Could you check a few things on this model? Use its own coordinates, in mm. Face numbers are marked on the shaded views. A direction names the side the tool comes from. Give positions to 0.01 mm unless a question says otherwise; leave off trailing zeros. Write each loop counter-clockwise with the first axis right and the second up, starting at its lowest first coordinate (ties: lowest second). Pieces come first, ordered by that corner, then holes. Notation, with made-up numbers: (-10.5, -14) - (0.5, -14) arc R31 ccw to (0.5, 21) - close; hole circle Ø1 at (-19, 7). An arc over 180 degrees is marked (long way). Answer as CSV lines item,"result". Start each with the question number.
Q1. On a 3-axis mill with a long thin cutter (end or side, diameter ignored), from which of +Z, -Z, +X, -X, +Y, -Y can I reach the whole of each face in a straight line? I mean the marked faces 1, 2 and 3. Say none if no direction works.
Q2. If I drill on line 1 along Y through (x, z) = (-13.75, 67.1); line 2 along X through (y, z) = (7, 43); line 3 along Z through (x, y) = (-3, -14.5), over which ranges is the centre line in solid material (lowest first)?
Q3. Imagine slicing it at C-C on y = -30.16. List the corners of the cut face in (x, z) for me, and give its area (3 significant figures).
Q4. Imagine slicing it at B-B on z = 67.1. List the corners of the cut face in (x, y) for me.
Q5. Will these pins go through, and if not, where does the flat tip stop? pin 1 Ø0.7 at (y, z) = (-14.5, 21) entering from +X; pin 2 Ø0.5 at (x, z) = (5, 0) entering from -Y; pin 3 Ø8 at (x, y) = (-2, -7.5) entering from +Z; pin 4 Ø2.5 at (y, z) = (2.34, 49.9) entering from -X.
Q6. Imagine slicing it at D-D on z = 30.5. List the corners of the cut face in (x, y) for me, and give its area (3 significant figures).
Q7. Imagine slicing it at A-A on y = 2.34. List the corners of the cut face in (x, z) for me.
```python
from build123d import *

# Parameters (mm, degrees)
SKETCH1_W                    = 28.1256
SKETCH1_H                    = 30
BASE_FLANGE2_DEPTH           = 0.8128
EDGE_FLANGE3_STRIP_W         = 4.7244
EDGE_FLANGE3_STRIP_H         = 0.8128
EDGE_FLANGE3_STRIP_CUT_DEPTH = 30
EDGE_FLANGE3_DEPTH           = 30
EDGE_FLANGE3_FLAT_DEPTH      = 0.8128
EDGE_FLANGE4_START           = 0.7366
EDGE_FLANGE4_DEPTH           = 56.7698
EDGE_FLANGE4_START_2         = 57.1
EDGE_FLANGE4_2_DEPTH         = 0.4064
EDGE_FLANGE4_3_DEPTH         = 56.3634
CUT_EXTRUDE1_REACH           = 93.299
SKETCH22_R                   = 2
CUT_EXTRUDE2_REACH           = 89.146


# Read off the part's stored shape, not the designer's step: Edge-Flange4
# Sheet-metal steps are written as plain solids
with BuildPart() as part:
    # Sketch1 → Base-Flange2 (new body)
    with BuildSketch(Plane.XY):
        Rectangle(SKETCH1_W, SKETCH1_H)
    extrude(amount=-BASE_FLANGE2_DEPTH)

    # Edge-Flange3 strip (across the edge) → Edge-Flange3 strip cut (cut)
    with BuildSketch(Plane(origin=(-14.0628, 15, 0), x_dir=(1, 0, 0), z_dir=(0, -1, 0))):
        with Locations((-0.8128, -0.4064)):
            Rectangle(EDGE_FLANGE3_STRIP_W, EDGE_FLANGE3_STRIP_H)
    extrude(amount=EDGE_FLANGE3_STRIP_CUT_DEPTH, mode=Mode.SUBTRACT)

    # Edge-Flange3 bend section (across the edge) → Edge-Flange3 (add)
    with BuildSketch(Plane(origin=(-14.0628, 15, 0), x_dir=(1, 0, 0), z_dir=(0, -1, 0))):
        with BuildLine():
            Line((0, 0.7366), (0.8128, 0.7366))
            ThreePointArc((0.8128, 0.7366), (1.028545145, 0.215745145), (1.5494, 0))
            Line((1.5494, 0), (1.5494, -0.8128))
            ThreePointArc((1.5494, -0.8128), (0.453808753, -0.358991247), (0, 0.7366))
        make_face()
    extrude(amount=EDGE_FLANGE3_DEPTH)

    # Edge-Flange3 profile (on flange) → Edge-Flange3 flat (add)
    with BuildSketch(Plane(origin=(-14.0628, 0, 0), x_dir=(0, -1, 0), z_dir=(-1, 0, 0))):
        Polygon((-15, 0.7366), (15, 0.7366), (15, 57.1), (40, 57.1), (40, 77.1), (-15, 77.1), align=None)
    extrude(amount=-EDGE_FLANGE3_FLAT_DEPTH)

    # Edge-Flange4 outline → Edge-Flange4 (cut)
    with BuildSketch(Plane.XY.offset(EDGE_FLANGE4_START)):
        with BuildLine():
            ThreePointArc((-13.25, -13.4506), (-13.468624211, -14.244121367), (-14.0628, -14.813707039))
            Line((-14.0628, -14.813707039), (-14.0628, -15))
            Line((-14.0628, -15), (-13.25, -15))
            Line((-13.25, -15), (-13.25, -13.4506))
        make_face()
    extrude(amount=EDGE_FLANGE4_DEPTH, mode=Mode.SUBTRACT)

    # Edge-Flange4 2 outline → Edge-Flange4 2 (cut)
    with BuildSketch(Plane.XY.offset(EDGE_FLANGE4_START_2)):
        with BuildLine():
            Line((-14.0628, -13.0442), (-14.0628, -14.813707039))
            ThreePointArc((-14.0628, -14.813707039), (-13.468624211, -14.244121367), (-13.25, -13.4506))
            Line((-13.25, -13.4506), (-13.25, -13.0442))
            Line((-13.25, -13.0442), (-14.0628, -13.0442))
        make_face()
    extrude(amount=EDGE_FLANGE4_2_DEPTH, mode=Mode.SUBTRACT)

    # Edge-Flange4 3 outline → Edge-Flange4 3 (add)
    with BuildSketch(Plane.XY.offset(EDGE_FLANGE4_START)):
        with BuildLine():
            Line((-28.25, -15), (-14.7994, -15))
            ThreePointArc((-14.7994, -15), (-14.419503755, -14.952704924), (-14.0628, -14.813707039))
            Line((-14.0628, -14.813707039), (-14.0628, -13.4506))
            ThreePointArc((-14.0628, -13.4506), (-14.278545145, -13.971454855), (-14.7994, -14.1872))
            Line((-14.7994, -14.1872), (-28.25, -14.1872))
            Line((-28.25, -14.1872), (-28.25, -15))
        make_face()
    extrude(amount=EDGE_FLANGE4_3_DEPTH)

    # Sketch22 → Cut-Extrude1 (cut, up to next)
    with BuildSketch(Plane.ZY.offset(14.0628), mode=Mode.PRIVATE) as cut_extrude1_sk1:
        with Locations((67.1, -30.16)):
            Circle(SKETCH22_R)
    cut_extrude1_tool1 = extrude(cut_extrude1_sk1.sketch, amount=-CUT_EXTRUDE1_REACH, mode=Mode.PRIVATE) & part.part
    # Sketch22 → Cut-Extrude1 (cut, up to next)
    with BuildSketch(Plane.ZY.offset(14.0628), mode=Mode.PRIVATE) as cut_extrude1_sk2:
        with Locations((67.1, -7.66)):
            Circle(SKETCH22_R)
    cut_extrude1_tool2 = extrude(cut_extrude1_sk2.sketch, amount=-CUT_EXTRUDE1_REACH, mode=Mode.PRIVATE) & part.part
    # Sketch22 → Cut-Extrude1 (cut, up to next)
    with BuildSketch(Plane.ZY.offset(14.0628), mode=Mode.PRIVATE) as cut_extrude1_sk3:
        with Locations((49.895058849, 2.34)):
            Circle(SKETCH22_R)
    cut_extrude1_tool3 = extrude(cut_extrude1_sk3.sketch, amount=-CUT_EXTRUDE1_REACH, mode=Mode.PRIVATE) & part.part
    # Sketch22 → Cut-Extrude1 (cut, up to next)
    with BuildSketch(Plane.ZY.offset(14.0628), mode=Mode.PRIVATE) as cut_extrude1_sk4:
        with Locations((29.995058849, 2.34)):
            Circle(SKETCH22_R)
    cut_extrude1_tool4 = extrude(cut_extrude1_sk4.sketch, amount=-CUT_EXTRUDE1_REACH, mode=Mode.PRIVATE) & part.part
    # Sketch22 → Cut-Extrude1 (cut, up to next)
    with BuildSketch(Plane.ZY.offset(14.0628), mode=Mode.PRIVATE) as cut_extrude1_sk5:
        with Locations((10.095058849, 2.34)):
            Circle(SKETCH22_R)
    cut_extrude1_tool5 = extrude(cut_extrude1_sk5.sketch, amount=-CUT_EXTRUDE1_REACH, mode=Mode.PRIVATE) & part.part
    add(cut_extrude1_tool1.solids().sort_by_distance((-14.0628, -30.16, 67.1))[0], mode=Mode.SUBTRACT)
    add(cut_extrude1_tool2.solids().sort_by_distance((-14.0628, -7.66, 67.1))[0], mode=Mode.SUBTRACT)
    add(cut_extrude1_tool3.solids().sort_by_distance((-14.0628, 2.34, 49.895059))[0], mode=Mode.SUBTRACT)
    add(cut_extrude1_tool4.solids().sort_by_distance((-14.0628, 2.34, 29.995059))[0], mode=Mode.SUBTRACT)
    add(cut_extrude1_tool5.solids().sort_by_distance((-14.0628, 2.34, 10.095059))[0], mode=Mode.SUBTRACT)

    # Sketch23 → Cut-Extrude2 (cut, up to next)
    with BuildSketch(Plane(origin=(0, -14.1872, 0), x_dir=(1, 0, 0), z_dir=(0, 1, 0)), mode=Mode.PRIVATE) as cut_extrude2_sk1:
        with BuildLine():
            Line((-26.8128, -26.4866), (-26.8128, -18.4866))
            ThreePointArc((-26.8128, -18.4866), (-24.0628, -15.7366), (-21.3128, -18.4866))
            Line((-21.3128, -18.4866), (-21.3128, -26.4866))
            ThreePointArc((-21.3128, -26.4866), (-24.0628, -29.2366), (-26.8128, -26.4866))
        make_face()
    cut_extrude2_tool1 = extrude(cut_extrude2_sk1.sketch, amount=-CUT_EXTRUDE2_REACH, mode=Mode.PRIVATE) & part.part
    # Sketch23 → Cut-Extrude2 (cut, up to next)
    with BuildSketch(Plane(origin=(0, -14.1872, 0), x_dir=(1, 0, 0), z_dir=(0, 1, 0)), mode=Mode.PRIVATE) as cut_extrude2_sk2:
        with BuildLine():
            Line((-26.8128, -41.9866), (-26.8128, -49.9866))
            ThreePointArc((-26.8128, -49.9866), (-24.0628, -52.7366), (-21.3128, -49.9866))
            Line((-21.3128, -49.9866), (-21.3128, -41.9866))
            ThreePointArc((-21.3128, -41.9866), (-24.0628, -39.2366), (-26.8128, -41.9866))
        make_face()
    cut_extrude2_tool2 = extrude(cut_extrude2_sk2.sketch, amount=-CUT_EXTRUDE2_REACH, mode=Mode.PRIVATE) & part.part
    add(cut_extrude2_tool1.solids().sort_by_distance((-24.0628, -14.1872, 22.4866))[0], mode=Mode.SUBTRACT)
    add(cut_extrude2_tool2.solids().sort_by_distance((-24.0628, -14.1872, 45.9866))[0], mode=Mode.SUBTRACT)


solid = part.part
```
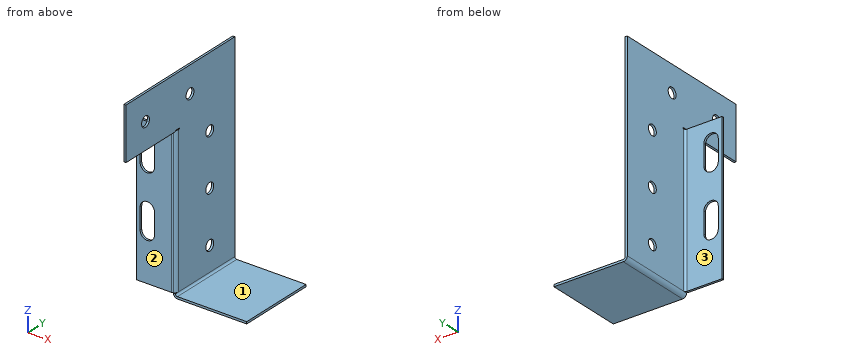
Conclusion:
1,face 1,"+Z, +X, +Y, -Y"
1,face 2,"+Z, -Z, +X, -X, -Y"
1,face 3,"+Z, -Z, -X, +Y"
2,line 1,"-40 to -32.16, -28.16 to -9.66, -5.66 to 15"
2,line 2,"-14.06 to -13.25"
2,line 3,"-0.81 to 0"
3,outline,"(-14.06, 57.1) - (-13.25, 57.1) - (-13.25, 65.1) - (-14.06, 65.1) - close; (-14.06, 69.1) - (-13.25, 69.1) - (-13.25, 77.1) - (-14.06, 77.1) - close"
3,area,"13.0 mm^2"
4,outline,"(-14.06, -40) - (-13.25, -40) - (-13.25, -32.16) - (-14.06, -32.16) - close; (-14.06, -28.16) - (-13.25, -28.16) - (-13.25, -9.66) - (-14.06, -9.66) - close; (-14.06, -5.66) - (-13.25, -5.66) - (-13.25, 15) - (-14.06, 15) - close"
5,pin 1,"x = -13.42"
5,pin 2,"y = -15"
5,pin 3,"z = 0"
5,pin 4,"through"
6,outline,"(-28.25, -15) - (-14.8, -15) arc R1.55 ccw to (-13.25, -13.45) - (-13.25, 0.4) - (-14.06, 0.4) - (-14.06, -13.45) arc R0.74 cw to (-14.8, -14.19) - (-28.25, -14.19) - close; (-14.06, 4.28) - (-13.25, 4.28) - (-13.25, 15) - (-14.06, 15) - close"
6,area,"32.4 mm^2"
7,outline,"(-14.06, 0.74) arc R1.55 ccw to (-12.51, -0.81) - (14.06, -0.81) - (14.06, 0) - (-12.51, 0) arc R0.74 cw to (-13.25, 0.74) - (-13.25, 8.1) - (-14.06, 8.1) - close; (-14.06, 12.1) - (-13.25, 12.1) - (-13.25, 28) - (-14.06, 28) - close; (-14.06, 32) - (-13.25, 32) - (-13.25, 47.9) - (-14.06, 47.9) - close; (-14.06, 51.9) - (-13.25, 51.9) - (-13.25, 77.1) - (-14.06, 77.1) - close"
